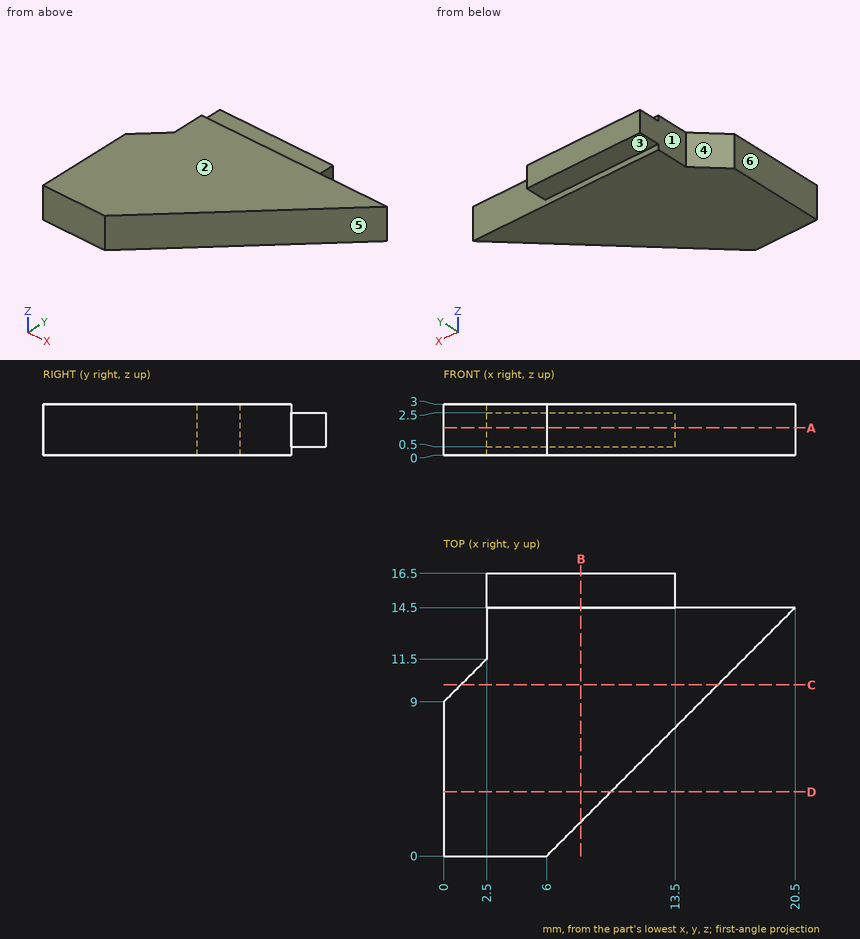
Verification items for this drawing (mm, ordinates from the low corner). A direction names the side the tool comes from. Give positions to 0.01 mm unless a question says otherwise; leave off trailing zeros. Write each loop counter-clockwise with the first axis right and the second up, starting at its lowest first coordinate (ties: lowest second). Pieces come first, ordered by that corner, then holes. Notation, with made-up numbers: (77, 75.25) -> (127, 75.25) arc R26 ccw to (127, 100.25) -> close; hole circle Ø9 at (4, 54). An arc over 180 degrees is marked (long way). Use CSV: the item, a comma, the result in double quotes. Start each with the question number.
Q1. Cross-section at A-A on z = 1.6. Enter the section's corners in (x, y).
Q2. Cross-section at B-B on x = 8. Enter the section's corners in (y, z).
Q3. Tool access check on the marked faces 1, 2 and 3. Record the directions out of +Z, -Z, +X, -X, +Y, -Y that give a thin tool (end or side, any length) a straight path to the whole face; none if there is none.
Q4. Cross-section at D-D on y = 3.75. Enter the section's corners in (x, z), and give its area (4 significant figures).
Q5. Depth check by flat-ended pin: P1, Ø1.6, axis at x = 10, y = 15.5, coming from the +Z side; P2, Ø0.9, axis at y = 15, z = 1.5, coming from the -X side. Enter the tip coordinate at first touch or a pass-through.
Q6. Cross-section at C-C on y = 10. Enter the section's corners in (x, z), and give its area (3 significant figures).
Q7. Scan lines: line 1 along Z through (x, y) = (7, 15); line 2 along Y through (x, z) = (4.5, 0.45); line 3 along X through (y, z) = (7.5, 0.5). Record each from-to range of solid material in increasing order.
Q8. Release check for a two-part mould opening along Y. For the marked faces 4, 5 and 6 record: +Y half, -Y half, draft (parallel to the pull), parting line (faces both ways), or undercut.
Working result:
1,outline,"(0, 0) -> (6, 0) -> (20.5, 14.5) -> (13.5, 14.5) -> (13.5, 16.5) -> (2.5, 16.5) -> (2.5, 11.5) -> (0, 9) -> close"
2,outline,"(2, 0) -> (14.5, 0) -> (14.5, 0.5) -> (16.5, 0.5) -> (16.5, 2.5) -> (14.5, 2.5) -> (14.5, 3) -> (2, 3) -> close"
3,face 1,"+Z, -Z, -X, +Y"
3,face 2,"+Z, +X, -X, +Y, -Y"
3,face 3,"-Z, +X, -X, +Y"
4,outline,"(0, 0) -> (9.75, 0) -> (9.75, 3) -> (0, 3) -> close"
4,area,"29.25 mm^2"
5,P1,"stops at z = 2.5"
5,P2,"stops at x = 2.5"
6,outline,"(1, 0) -> (16, 0) -> (16, 3) -> (1, 3) -> close"
6,area,"45.0 mm^2"
7,line 1,"z = 0.5 to 2.5"
7,line 2,"y = 0 to 14.5"
7,line 3,"x = 0 to 13.5"
8,face 4,"+Y half"
8,face 5,"-Y half"
8,face 6,"draft"
